```python
from build123d import *

# Parameters (mm, degrees)
PAD_DEPTH = 10
FILLET_R  = 5


with BuildPart() as part:
    # Sketch → Pad (new body)
    with BuildSketch(Plane.XY):
        Polygon((0, 0), (-70, 0), (-95, -10), (-167, -10), (-167, 5), (-187, 5), (-187, 180), (-175, 180), (-175, 250), (0, 250), (175, 250), (175, 180), (187, 180), (187, 5), (167, 5), (167, -10), (95, -10), (70, 0), align=None)
    extrude(amount=PAD_DEPTH)

    # Fillet
    fillet_edges = [part.edges().sort_by_distance(p)[0] for p in [
        (-70, 0, 5),
        (70, 0, 5),
        (95, -10, 5),
        (167, -10, 5),
        (167, 5, 5),
        (187, 5, 5),
        (187, 180, 5),
        (175, 250, 5),
        (175, 180, 5),
        (-175, 250, 5),
        (-175, 180, 5),
        (-187, 180, 5),
        (-187, 5, 5),
        (-167, 5, 5),
        (-167, -10, 5),
        (-95, -10, 5),
    ]]
    fillet(fillet_edges, radius=FILLET_R)


solid = part.part
```
Could you check a few things on this model? Use its own coordinates, in mm. A direction names the side the tool comes from. Round coordinates to 2 decimals unless told otherwise and drop trailing zeros. Order: outer loops, then holes, each group sorted by start corner. A loop starts at its lowest first (then second) coordinate and runs counter-clockwise, first axis right, second up. Notation, with made-up numbers: (-33.5, 81.25) -> (-3.5, 81.25) arc R21 cw to (-3.5, 118.25) -> close; hole circle Ø5 at (65, -34.5). An arc over 180 degrees is marked (long way). One line per question, with ' | ' between items.
Q1. If we section it at B-B on x = -58.5: Write out the boundary of the cut face in (y, z).
Computed values:
outline: (0, 0) -> (250, 0) -> (250, 10) -> (0, 10) -> close
Q2. If we section it at C-C on y = 224.5: Write out the boundary of the cut face in (x, z), plus the area to 3 significant figures.
Computed values:
outline: (-175, 0) -> (175, 0) -> (175, 10) -> (-175, 10) -> close | area: 3,500 mm²
Q3. If I drill on line 1 (X direction, y = 194, z = 5); line 2 (Y direction, x = 67, z = 0.5); line 3 (Y direction, x = 74.5, z = 6), over which ranges is the centre line in solid material (lowest first)? Write a range as from..to.
Computed values:
line 1: -175..175 | line 2: 0..250 | line 3: -1.8..250
Q4. I'm going to push flat-ended pins straight in: pin 1 (4 mm diameter, centred on y = 192, z = 8.5, fed in from +X); pin 2 (1 mm diameter, centred on x = 181, z = 3, fed in from +Y); pin 3 (5.5 mm diameter, centred on y = -3, z = 5, fed in from -X). Where does each tip first touch, or does it pass through?
Computed values:
pin 1: x = 175 | pin 2: y = 180 | pin 3: x = -167
Q5. Which directions (+Z, -Z, +X, -X, +Y, -Y) give clear straight access to the entire face, cutting with the end or side of a thin tool? Please do faces 5 (the face through (-129, -10, 5)), 6 (the face through (-175, 215, 5)), 7 (the face through (-82.338, -4.935, 4.93)), 8 (the face through (177, 5, 5)), 9 (the face through (-177, 5, 5)).
Computed values:
face 5: +Z, -Z, +X, -X, -Y | face 6: +Z, -Z, -X, +Y | face 7: +Z, -Z, -Y | face 8: +Z, -Z, +X, -Y | face 9: +Z, -Z, -X, -Y
Q6. We'd pull the mould along X, two halves only. Please class faces 1 (the face through (3, 122, 0)), 2 (the face through (-1, 0, 5)), 3 (the face through (82.662, -5.065, 4.93)), 4 (the face through (175, 215, 5)): released by +X, released by -X, zero draft, split by the parting line, or undercut.
Computed values:
face 1: zero draft | face 2: undercut | face 3: undercut | face 4: released by +X
